Part model, mm, in its own coordinate system. A direction names the side the tool comes from. Give positions to 0.01 mm unless a question says otherwise; leave off trailing zeros. Order: outer loops, then holes, each group sorted by start corner. A loop starts at its lowest first (then second) coordinate and runs counter-clockwise, first axis right, second up. Notation, with made-up numbers: (11.5, 53.5) - (39.5, 53.5) arc R13 ccw to (39.5, 77.5) - close; hole circle Ø9 at (85.25, 80). An arc over 180 degrees is marked (long way). One line per item, written item: value.
```python
from build123d import *

# Parameters (mm, degrees)
F1_W           = 76.2
F1_H           = 76.2
F1_W_2         = 63.5
F1_H_2         = 63.5
F3_W           = 76.2
F3_H           = 76.2
F3_W_2         = 63.5
F3_H_2         = 63.5
F4_DEPTH       = 800.1
F4_DEPTH_BACK  = 800.1
F5_W           = 25.4
F5_H           = 25.4
F5_W_2         = 19.05
F5_H_2         = 19.05
F6_DEPTH       = 793.75
F7_W           = 6.35
F7_H           = 25.4
F8_DEPTH       = 25.4
F9_W           = 1600.2
F9_H           = 2.667
F10_DEPTH      = 660.4
F10_DEPTH_BACK = 654.05
F11_R          = 11.1125
F12_DEPTH      = 101.601
F13_R          = 9.525
F14_DEPTH      = 76.2
F15_R          = 6.35
F16_DEPTH      = 241.3
F16_DEPTH_BACK = 101.6


# Not quite as in the source:
# - an extrude ends at something that could not be found from the text; its depth is read off the source's solid


with BuildPart() as f2:
    # F2: sweep along a path in F0
    with BuildLine(Plane.XZ) as f2_path:
        Line((-876.3, 660.4), (876.3, 660.4))
        Line((876.3, 660.4), (876.3, -654.05))
        Line((876.3, -654.05), (-876.3, -654.05))
        Line((-876.3, -654.05), (-876.3, 660.4))
    # F1 (on Top) → F2 (sweep)
    with BuildSketch(Plane.XY):
        with Locations((-838.2, -38.1)):
            Rectangle(F1_W, F1_H)
        with Locations((-838.2, -38.1)):
            Rectangle(F1_W_2, F1_H_2, mode=Mode.SUBTRACT)
    sweep(path=f2_path.line, transition=Transition.RIGHT)

    # F3 (on Right) → F4 (join, two sides)
    with BuildSketch(Plane.YZ) as f4_sk:
        with Locations((-38.1, 279.4)):
            Rectangle(F3_W, F3_H)
        with Locations((-38.1, 279.4)):
            Rectangle(F3_W_2, F3_H_2, mode=Mode.SUBTRACT)
        with Locations((-38.1, -139.7)):
            Rectangle(F3_W, F3_H)
        with Locations((-38.1, -139.7)):
            Rectangle(F3_W_2, F3_H_2, mode=Mode.SUBTRACT)
    extrude(amount=-F4_DEPTH)
    extrude(f4_sk.sketch, amount=F4_DEPTH_BACK)

    # F5 (on Right) → F6 (join, symmetric)
    with BuildSketch(Plane.YZ):
        with Locations((-88.9, -139.7)):
            Rectangle(F5_W, F5_H)
        with Locations((-88.9, -139.7)):
            Rectangle(F5_W_2, F5_H_2, mode=Mode.SUBTRACT)
    extrude(amount=F6_DEPTH, both=True)

    # F7 (on face) → F8 (join, through all)
    with BuildSketch(Plane.XY.offset(-127)):
        with Locations((790.575, -88.9)):
            Rectangle(F7_W, F7_H)
        with Locations((-790.575, -88.9)):
            Rectangle(F7_W, F7_H)
    extrude(amount=-F8_DEPTH)

    # F9 (on Top) → F10 (join, two sides)
    with BuildSketch(Plane.XY) as f10_sk:
        with Locations((0, -74.8665)):
            Rectangle(F9_W, F9_H)
    extrude(amount=F10_DEPTH)
    extrude(f10_sk.sketch, amount=-F10_DEPTH_BACK)

    # F11 (on Front) → F12 (cut, through all)
    with BuildSketch(Plane.XZ):
        with Locations((-838.2, 514.35)):
            Circle(F11_R)
        with Locations((-838.2, 79.375)):
            Circle(F11_R)
        with Locations((-838.2, -355.6)):
            Circle(F11_R)
    extrude(amount=F12_DEPTH, mode=Mode.SUBTRACT)

    # F13 (on face) → F14 (cut, through all)
    with BuildSketch(Plane.XY.offset(317.5)):
        with Locations((-723.9, -38.1)):
            Circle(F13_R)
        with Locations((723.9, -38.1)):
            Circle(F13_R)
    extrude(amount=-F14_DEPTH, mode=Mode.SUBTRACT)

    # F15 (on Top) → F16 (join, two sides)
    with BuildSketch(Plane.XY) as f16_sk:
        with Locations((-647.7, -12.7)):
            Circle(F15_R)
    extrude(amount=F16_DEPTH)
    extrude(f16_sk.sketch, amount=-F16_DEPTH_BACK)


solid = f2.part
```
1) Cut at B-B, the plane z = 443.5. Give the cut face in (x, y).
Outcome:
outline: (-876.3, -76.2) - (876.3, -76.2) - (876.3, 0) - (800.1, 0) - (800.1, -73.53) - (-800.1, -73.53) - (-800.1, 0) - (-876.3, 0) - close; hole (-869.95, -69.85) - (-806.45, -69.85) - (-806.45, -6.35) - (-869.95, -6.35) - close; hole (806.45, -69.85) - (869.95, -69.85) - (869.95, -6.35) - (806.45, -6.35) - close
2) Cut at A-A, the plane z = 23. Give the cut face in (x, y), then the cut area to 3 significant figures.
Outcome:
outline: (-876.3, -76.2) - (876.3, -76.2) - (876.3, 0) - (800.1, 0) - (800.1, -73.53) - (-800.1, -73.53) - (-800.1, 0) - (-876.3, 0) - close; circle Ø12.7 at (-647.7, -12.7); hole (-869.95, -69.85) - (-806.45, -69.85) - (-806.45, -6.35) - (-869.95, -6.35) - close; hole (806.45, -69.85) - (869.95, -69.85) - (869.95, -6.35) - (806.45, -6.35) - close
area: 7,940 mm^2
3) Cut at D-D, the plane x = 521. Give the number of separate pieces and of enclosed holes in the cut face, then the cut area to 3 significant figures.
Outcome:
separate pieces: 1
enclosed holes: 5
area: 10,100 mm^2
4) Cut at C-C, the plane z = 289. Give the cut face in (x, y), then the cut area to 3 significant figures.
Outcome:
outline: (-876.3, -76.2) - (876.3, -76.2) - (876.3, 0) - (-876.3, 0) - close; hole (-869.95, -69.85) - (-806.45, -69.85) - (-806.45, -6.35) - (-869.95, -6.35) - close; hole (-800.1, -69.85) - (800.1, -69.85) - (800.1, -6.35) - (-800.1, -6.35) - close; hole (806.45, -69.85) - (869.95, -69.85) - (869.95, -6.35) - (806.45, -6.35) - close
area: 23,900 mm^2
5) Pin check, flat tips, straight feed: pin 1 (10 mm diameter, centred on x = -14, z = 433.5, fed in from -Y); pin 2 (21 mm diameter, centred on x = -98.5, y = -90.5, fed in from +Z); pin 3 (12.5 mm diameter, centred on x = -304, y = -89, fed in from -Z). Stop position of each tip, or through.
Outcome:
pin 1: stops at y = -76.2
pin 2: stops at z = -127
pin 3: stops at z = -152.4
6) Drill centre lines: line 1 along X through (y, z) = (-53, 171); line 2 along Z through (x, y) = (-838.2, -73.5); line 3 along Z through (x, y) = (-184, -4). Where is each one in solid material? Low to high. Write a range as from..to.
Outcome:
line 1: x = -876.3..-869.95, -806.45..-800.1, 800.1..806.45, 869.95..876.3
line 2: z = -654.05..-366.71, -344.49..68.26, 90.49..503.24, 525.46..660.4
line 3: z = -654.05..-577.85, -177.8..-101.6, 241.3..317.5, 584.2..660.4
7) Which spindle directions (+Z, -Z, +X, -X, +Y, -Y) get a long thin tool onto all of the face, cutting with end or side? Do faces 4 (the flat face through (-800.1, -39, 280)), 5 (the flat face through (-11, -37, -577.85)). Say none if no direction does.
Outcome:
face 4: none
face 5: +Y
8) Mould opens along Y. For faces 1 (the flat face through (800.1, -37, -381)), 2 (the flat face through (-11, -39, 247.65)), 3 (the flat face through (126, 0, -146)) say: released by +Y, released by -Y, zero draft, split by the parting line, or undercut.
Outcome:
face 1: zero draft
face 2: undercut
face 3: released by +Y
